The listing builds one solid part. Answer for the finished solid, in the listing's coordinates (mm). Face numbers are marked on the shaded views. Round coordinates to 2 decimals unless told otherwise and drop trailing zeros. Write each loop counter-clockwise with the first axis right and the second up, starting at its lowest first coordinate (ties: lowest second). Pieces come first, ordered by that corner, then holes. Notation, with made-up numbers: (-28.75, 67.25) - (-8.75, 67.25) arc R26 cw to (-8.75, 94.25) - close; hole circle Ø1 at (-24.5, -18.5). An arc over 180 degrees is marked (long way). Answer in a Markdown table with one row per item.
from build123d import *

# Parameters (mm, degrees)
F0_R        = 19.05
F1_DEPTH    = 127
F2_T        = -0.635
F3_W        = 10.16
F3_H        = 50.8
F3_H_2      = 127
F4_DEPTH    = 38.1
F5_T1_DEPTH = 127.6597299865
F5_T3_DEPTH = 127.6597299858
F5_T5_DEPTH = 127.6597299858
F5_T7_DEPTH = 127.6597299865


# Not quite as in the source:
# - a fillet or chamfer that OpenCascade refuses, or shapes differently, is made with other operations: its cross-section is extruded or revolved along the edge and cut away or added


with BuildPart() as f1:
    # F0 (on Top) → F1 (new body)
    with BuildSketch(Plane.XY):
        Circle(F0_R)
    extrude(amount=F1_DEPTH)

    # F2
    f2_openings = [f1.faces().sort_by_distance(p)[0] for p in [
        (0, 0, 0),
        (0, 0, 127),
    ]]
    offset(amount=F2_T, openings=f2_openings)

    # F3 (on Front) → F4 (cut, symmetric)
    with BuildSketch(Plane.XZ):
        with Locations((0, 50.8)):
            Rectangle(F3_W, F3_H)
        with Locations((-3.17e-08, 114.3)):
            Rectangle(F3_W, F3_H)
        with Locations((-0.4444076066, 213.36)):
            Rectangle(F3_W, F3_H_2)
    extrude(amount=F4_DEPTH, both=True, mode=Mode.SUBTRACT)

    # F5: fillet of radius 25.4 on 4 edges, made by hand

    # F5_s2 → F5_t1 (cut)
    with BuildSketch(Plane.XZ.offset(-45.7995529809)):
        with BuildLine():
            ThreePointArc((-5.0800000317, 101.6), (-12.5194877896, 119.5605122421), (-30.4800000317, 127))
            Line((-30.4800000317, 127), (-5.0800000317, 127))
            Line((-5.0800000317, 127), (-5.0800000317, 101.6))
        make_face()
    extrude(amount=F5_T1_DEPTH, mode=Mode.SUBTRACT)

    # F5_s4 → F5_t3 (cut)
    with BuildSketch(Plane.XZ.offset(-45.7995529626)):
        with BuildLine():
            ThreePointArc((30.4799999683, 127), (12.5194877261, 119.5605122421), (5.0799999683, 101.6))
            Line((5.0799999683, 101.6), (5.0799999683, 127))
            Line((5.0799999683, 127), (30.4799999683, 127))
        make_face()
    extrude(amount=F5_T3_DEPTH, mode=Mode.SUBTRACT)

    # F5_s6 → F5_t5 (cut)
    with BuildSketch(Plane.XZ.offset(-81.8601770232)):
        with BuildLine():
            ThreePointArc((30.4799999683, 127), (12.5194877261, 119.5605122421), (5.0799999683, 101.6))
            Line((5.0799999683, 101.6), (5.0799999683, 127))
            Line((5.0799999683, 127), (30.4799999683, 127))
        make_face()
    extrude(amount=F5_T5_DEPTH, mode=Mode.SUBTRACT)

    # F5_s8 → F5_t7 (cut)
    with BuildSketch(Plane.XZ.offset(-81.8601770056)):
        with BuildLine():
            ThreePointArc((-30.4800000317, 127), (-12.5194877896, 119.5605122421), (-5.0800000317, 101.6))
            Line((-5.0800000317, 101.6), (-5.0800000317, 127))
            Line((-5.0800000317, 127), (-30.4800000317, 127))
        make_face()
    extrude(amount=F5_T7_DEPTH, mode=Mode.SUBTRACT)


solid = f1.part
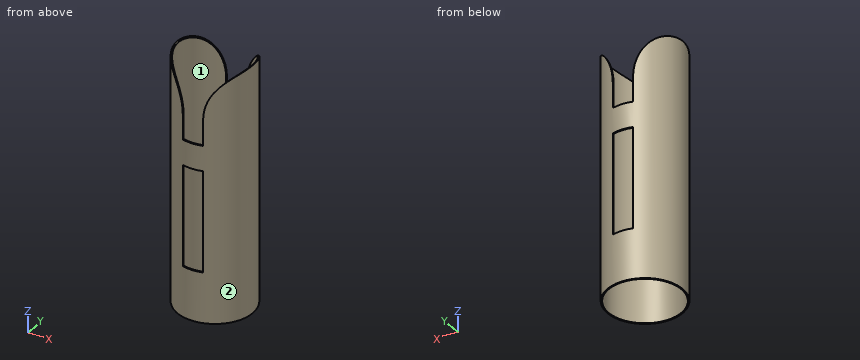
(1) Section C-C (x = 0) is taken. Give the vertices of the cut face in (y, z) (3 decimals).
Checked values:
| item | result |
|---|---|
| outline | (-19.05, 0) - (-18.415, 0) - (-18.415, 25.4) - (-19.05, 25.4) - close; (-19.05, 76.2) - (-18.415, 76.2) - (-18.415, 88.9) - (-19.05, 88.9) - close; (18.415, 0) - (19.05, 0) - (19.05, 25.4) - (18.415, 25.4) - close; (18.415, 76.2) - (19.05, 76.2) - (19.05, 88.9) - (18.415, 88.9) - close |
(2) Section A-A (z = 92.5) is taken. Give the vertices of the cut face in (x, y) (3 decimals), and give its area (3 significant figures).
Checked values:
| item | result |
|---|---|
| outline | (-5.08, -18.36) - (-5.08, -17.7) arc R18.415 cw to (-5.08, 17.7) - (-5.08, 18.36) arc R19.05 ccw to start; (5.08, -18.36) arc R19.05 ccw to (5.08, 18.36) - (5.08, 17.7) arc R18.415 cw to (5.08, -17.7) - close |
| area | 61.7 mm2 |
(3) Flat-ended cylindrical pins translate along their axes: pin 1 (10 mm diameter, centred on x = -15, z = 90.5, fed in from -Y); pin 2 (0.7 mm diameter, centred on x = 0.5, y = -18.5, fed in from +Z); pin 3 (0.7 mm diameter, centred on y = -18, z = 44.5, fed in from +X). Find the tip coordinate at first contact, or state that the pin passes through.
Checked values:
| item | result |
|---|---|
| pin 1 | stops at y = -16.21 |
| pin 2 | stops at z = 88.9 |
| pin 3 | stops at x = 7.17 |
(4) Section D-D (z = 16) is taken. Give the vertices of the cut face in (x, y) (3 decimals).
Checked values:
| item | result |
|---|---|
| outline | circle Ø38.1 at (0, 0); hole circle Ø36.83 at (0, 0) |
(5) Find the intervals of material crossed by line 1 (Y direction, x = 0, z = 77.5) (3 decimals); line 2 (Y direction, x = -17, z = 107.5), in increasing order.
Checked values:
| item | result |
|---|---|
| line 1 | y = -19.05 to -18.415, 18.415 to 19.05 |
| line 2 | y = -8.6 to -7.08, 7.08 to 8.6 |
(6) Section B-B (y = 0) is taken. Give the vertices of the cut face in (x, z) (3 decimals), and give its area (3 significant figures).
Checked values:
| item | result |
|---|---|
| outline | (-19.05, 0) - (-18.415, 0) - (-18.415, 123.952) arc R25.4 ccw to (-19.05, 124.283) - close; (18.415, 0) - (19.05, 0) - (19.05, 124.283) arc R25.4 ccw to (18.415, 123.952) - close |
| area | 158 mm2 |
(7) For a pull along X with two mould halves and no side action, classify the marked faces 1 and 2 as pulls with the +X half, pulls with the -X half, needs draft (parallel to the pull), parting line crosses it, or undercut.
Checked values:
| item | result |
|---|---|
| face 1 | undercut |
| face 2 | parting line crosses it |
